Part model, mm, in its own coordinate system. A direction names the side the tool comes from. Round coordinates to 2 decimals unless told otherwise and drop trailing zeros. Loops run counter-clockwise (first coordinate to the right, second up) from the corner with the lowest first, then second, coordinate; pieces in that order, holes last. Notation, with made-up numbers: (8, -12) - (28, -12) arc R18 ccw to (28, 1) - close; hole circle Ø1 at (30.5, 58). An arc over 180 degrees is marked (long way). Put each result on its own line as item: value.
from build123d import *

# Parameters (mm, degrees)
F1_DEPTH = 38.1
F2_R     = 1.9304
F3_DEPTH = 50.8
F4_R     = 1.27


with BuildPart() as f1:
    # F0 (on Top) → F1 (new body)
    with BuildSketch(Plane.XY):
        Polygon((-1.570657, -2.248221), (-14.905657, -37.808221), (11.764343, -37.808221), align=None)
    extrude(amount=F1_DEPTH)

    # F2 (on Top) → F3 (join)
    with BuildSketch(Plane.XY):
        with Locations((-2.001594, -24.78213)):
            Circle(F2_R)
    extrude(amount=F3_DEPTH)

    # F4
    f4_edges = [f1.edges().sort_by_distance(p)[0] for p in [
        (-1.570657, -2.248221, 19.05),
        (11.764343, -37.808221, 19.05),
        (-14.905657, -37.808221, 19.05),
        (-1.570657, -37.808221, 38.1),
        (5.096843, -20.028221, 38.1),
        (-8.238157, -20.028221, 38.1),
        (5.096843, -20.028221, 0),
        (-8.238157, -20.028221, 0),
        (-1.570657, -37.808221, 0),
    ]]
    fillet(f4_edges, radius=F4_R)


solid = f1.part
1. Tool access for faces 1 (the cylindrical face through (-14.127, -37.247, 19.299)), 2 (the cylindrical face through (-2.42, -26.667, 44.361)): list every direction of +Z, -Z, +X, -X, +Y, -Y with a clear straight run to the whole face (end or side of a thin tool).
A:
face 1: +Z, -Z, -X
face 2: +Z
2. Band-saw the part on A-A (z = 4.5). List the corners of the cut face in (x, y), plus the area to 3 significant figures.
A:
outline: (-14.26, -36.09) arc R1.27 ccw to (-13.07, -37.81) - (9.93, -37.81) arc R1.27 ccw to (11.12, -36.09) - (-0.38, -5.42) arc R1.27 ccw to (-2.76, -5.42) - close
area: 470 mm²
3. Pin check, flat tip, straight feed: P1, Ø10, axis at x = 8.5, y = -18.5, coming from the +Z side. Stop position of the tip, or through.
A:
P1: stops at z = 38.1
4. Probe line 1 along Z through (x, y) = (-3, -18); line 2 along X through (y, z) = (-23, 15); line 3 along Z through (x, y) = (9.5, -33.5). List the from-to ranges inside material, lowest first. Write a range as [from, to].
A:
line 1: z = [0, 38.1]
line 2: x = [-9.35, 6.21]
line 3: z = [0.19, 37.91]
